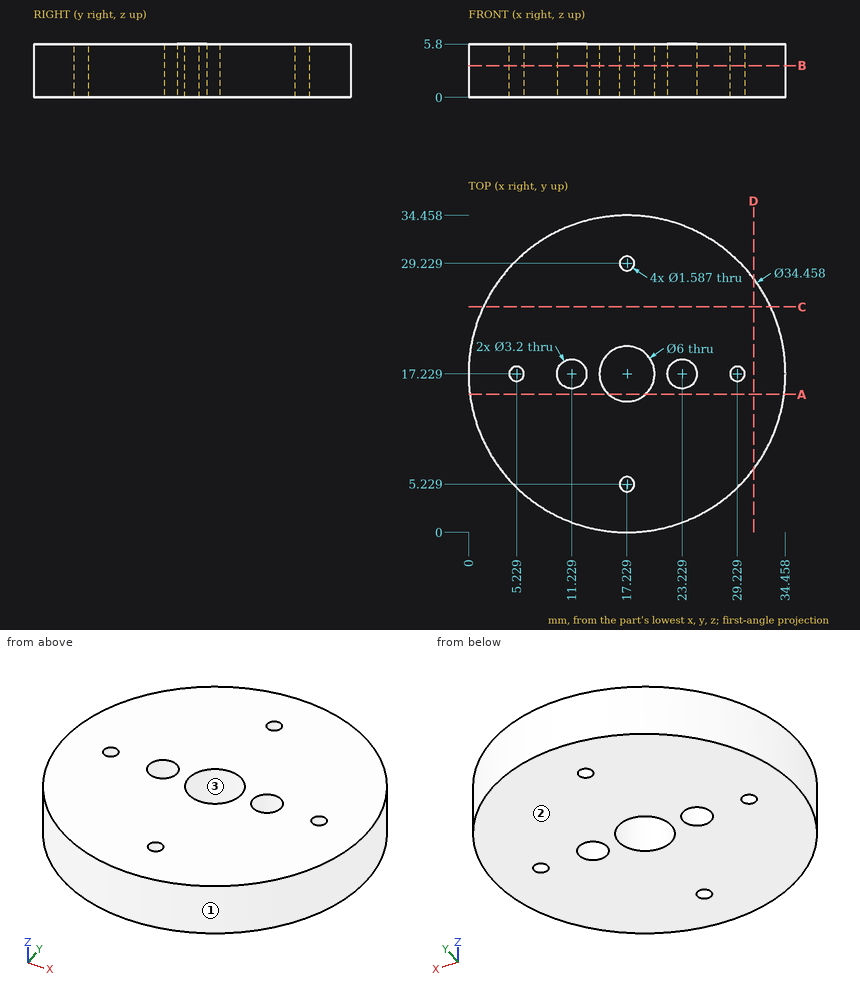
Could you check a few things on this drawing? It's one solid part, dimensions in mm from its lowest x, y, z. Give positions to 0.01 mm unless a question says otherwise; leave off trailing zeros. Order: outer loops, then holes, each group sorted by start corner. A loop starts at its lowest first (then second) coordinate and runs counter-clockwise, first axis right, second up. Notation, with made-up numbers: M 16.25,85.5 L 38.25,85.5 A27 ccw 38.25,102.5 Z; hole C 47,68.5 d11. An arc over 180 degrees is marked long. Use one line per item in the form item = value.
Item 1: If we section it at B-B, the plane z = 3.45: Write out the boundary of the cut face in (x, y).
Values follow:
outline = C 17.23,17.23 d34.46; hole C 5.23,17.23 d1.59; hole C 11.23,17.23 d3.2; hole C 17.23,17.23 d6; hole C 17.23,5.23 d1.59; hole C 17.23,29.23 d1.59; hole C 23.23,17.23 d3.2; hole C 29.23,17.23 d1.59
Item 2: If we section it at C-C, the plane y = 24.5: Write out the boundary of the cut face in (x, z), and give its area (3 significant figures).
Values follow:
outline = M 1.61,0 L 32.85,0 L 32.85,5.8 L 1.61,5.8 Z
area = 181 mm^2
Item 3: Will these pins go through, and if not, where does the flat tip stop? pin 1 Ø1 at (x, y) = (29.23, 17.23) entering from -Z; pin 2 Ø1 at (x, z) = (24.5, 4.5) entering from -Y; pin 3 Ø2 at (x, z) = (7, 3) entering from +Y; pin 4 Ø1.5 at (x, z) = (6, 3.5) entering from +Y (1 decimal).
Values follow:
pin_1 = through
pin_2 = 1.39
pin_3 = 31.78
pin_4 = 30.9
Item 4: If we section it at D-D, the plane x = 31: Write out the boundary of the cut face in (y, z) (1 decimal).
Values follow:
outline = M 6.9,0 L 27.6,0 L 27.6,5.8 L 6.9,5.8 Z
Item 5: If I drill on line 1 along Y through (x, z) = (11.5, 3.8) (1 decimal); line 2 along X through (y, z) = (3.5, 2.6) (1 decimal); line 3 along X through (y, z) = (10, 4.6), over which ranges is the centre line in solid material (lowest first)? Write a range as [from, to].
Values follow:
line_1 = [1, 15.7], [18.8, 33.5]
line_2 = [6.8, 27.6]
line_3 = [1.59, 32.87]
Item 6: Thinking about a two-plate mould opening in Y: for the marked faces 1, 2 and 3, which applies, pulls with the +Y half, pulls with the -Y half, needs draft (parallel to the pull), parting line crosses it, or undercut?
Values follow:
face_1 = parting line crosses it
face_2 = needs draft
face_3 = undercut
Item 7: If we section it at A-A, the plane y = 15: Write out the boundary of the cut face in (x, z) (1 decimal), and give its area (3 significant figures).
Values follow:
outline = M 0.1,0 L 15.2,0 L 15.2,5.8 L 0.1,5.8 Z; M 19.2,0 L 34.3,0 L 34.3,5.8 L 19.2,5.8 Z
area = 175 mm^2
